Check sheet for the modelled part. Datum: model origin and axes. Units: mm. Round coordinates to 2 decimals unless told otherwise and drop trailing zeros. Answer in a Markdown table with one row per item.
from build123d import *

# Parameters (mm, degrees)
SKETCH_1_W      = 1.6
SKETCH_1_H      = 5.6
SKETCH_1_W_2    = 1.25
EXTRUDE_1_DEPTH = 100


with BuildPart() as part:
    # 草图1 → 凸台-拉伸1 (new body)
    with BuildSketch(Plane.XY):
        Polygon((-63.5, 1.710790235), (-63.5, -0.999209765), (63.5, -0.999209765), (63.5, 1.710790235), (61.9, 1.710790235), (59.4, 1.710790235), (58.15, 1.710790235), (56.03, 1.710790235), (54.78, 1.710790235), (52.66, 1.710790235), (51.41, 1.710790235), (49.29, 1.710790235), (48.04, 1.710790235), (45.92, 1.710790235), (44.67, 1.710790235), (42.55, 1.710790235), (41.3, 1.710790235), (39.18, 1.710790235), (37.93, 1.710790235), (35.81, 1.710790235), (34.56, 1.710790235), (32.44, 1.710790235), (31.19, 1.710790235), (29.07, 1.710790235), (27.82, 1.710790235), (25.7, 1.710790235), (24.45, 1.710790235), (22.33, 1.710790235), (21.08, 1.710790235), (18.96, 1.710790235), (17.71, 1.710790235), (15.59, 1.710790235), (14.34, 1.710790235), (12.22, 1.710790235), (10.97, 1.710790235), (8.85, 1.710790235), (7.6, 1.710790235), (5.48, 1.710790235), (4.23, 1.710790235), (2.11, 1.710790235), (0.86, 1.710790235), (-1.26, 1.710790235), (-2.51, 1.710790235), (-4.63, 1.710790235), (-5.88, 1.710790235), (-8, 1.710790235), (-9.25, 1.710790235), (-11.37, 1.710790235), (-12.62, 1.710790235), (-14.74, 1.710790235), (-15.99, 1.710790235), (-18.11, 1.710790235), (-19.36, 1.710790235), (-21.48, 1.710790235), (-22.73, 1.710790235), (-24.85, 1.710790235), (-26.1, 1.710790235), (-28.22, 1.710790235), (-29.47, 1.710790235), (-31.59, 1.710790235), (-32.84, 1.710790235), (-34.96, 1.710790235), (-36.21, 1.710790235), (-38.33, 1.710790235), (-39.58, 1.710790235), (-41.7, 1.710790235), (-42.95, 1.710790235), (-45.07, 1.710790235), (-46.32, 1.710790235), (-48.44, 1.710790235), (-49.69, 1.710790235), (-51.81, 1.710790235), (-53.06, 1.710790235), (-55.18, 1.710790235), (-56.43, 1.710790235), (-58.55, 1.710790235), (-59.8, 1.710790235), (-61.9, 1.710790235), align=None)
        with Locations((-62.7, 4.510790235)):
            Rectangle(SKETCH_1_W, SKETCH_1_H)
        with Locations((62.7, 4.510790235)):
            Rectangle(SKETCH_1_W, SKETCH_1_H)
        with Locations((-59.175, 4.510790235)):
            Rectangle(SKETCH_1_W_2, SKETCH_1_H)
        with Locations((58.775, 4.510790235)):
            Rectangle(SKETCH_1_W_2, SKETCH_1_H)
        with Locations((-55.805, 4.510790235)):
            Rectangle(SKETCH_1_W_2, SKETCH_1_H)
        with Locations((55.405, 4.510790235)):
            Rectangle(SKETCH_1_W_2, SKETCH_1_H)
        with Locations((-52.435, 4.510790235)):
            Rectangle(SKETCH_1_W_2, SKETCH_1_H)
        with Locations((52.035, 4.510790235)):
            Rectangle(SKETCH_1_W_2, SKETCH_1_H)
        with Locations((-49.065, 4.510790235)):
            Rectangle(SKETCH_1_W_2, SKETCH_1_H)
        with Locations((48.665, 4.510790235)):
            Rectangle(SKETCH_1_W_2, SKETCH_1_H)
        with Locations((-45.695, 4.510790235)):
            Rectangle(SKETCH_1_W_2, SKETCH_1_H)
        with Locations((45.295, 4.510790235)):
            Rectangle(SKETCH_1_W_2, SKETCH_1_H)
        with Locations((-42.325, 4.510790235)):
            Rectangle(SKETCH_1_W_2, SKETCH_1_H)
        with Locations((41.925, 4.510790235)):
            Rectangle(SKETCH_1_W_2, SKETCH_1_H)
        with Locations((-38.955, 4.510790235)):
            Rectangle(SKETCH_1_W_2, SKETCH_1_H)
        with Locations((38.555, 4.510790235)):
            Rectangle(SKETCH_1_W_2, SKETCH_1_H)
        with Locations((-35.585, 4.510790235)):
            Rectangle(SKETCH_1_W_2, SKETCH_1_H)
        with Locations((35.185, 4.510790235)):
            Rectangle(SKETCH_1_W_2, SKETCH_1_H)
        with Locations((-32.215, 4.510790235)):
            Rectangle(SKETCH_1_W_2, SKETCH_1_H)
        with Locations((31.815, 4.510790235)):
            Rectangle(SKETCH_1_W_2, SKETCH_1_H)
        with Locations((-28.845, 4.510790235)):
            Rectangle(SKETCH_1_W_2, SKETCH_1_H)
        with Locations((28.445, 4.510790235)):
            Rectangle(SKETCH_1_W_2, SKETCH_1_H)
        with Locations((-25.475, 4.510790235)):
            Rectangle(SKETCH_1_W_2, SKETCH_1_H)
        with Locations((25.075, 4.510790235)):
            Rectangle(SKETCH_1_W_2, SKETCH_1_H)
        with Locations((-22.105, 4.510790235)):
            Rectangle(SKETCH_1_W_2, SKETCH_1_H)
        with Locations((21.705, 4.510790235)):
            Rectangle(SKETCH_1_W_2, SKETCH_1_H)
        with Locations((-18.735, 4.510790235)):
            Rectangle(SKETCH_1_W_2, SKETCH_1_H)
        with Locations((18.335, 4.510790235)):
            Rectangle(SKETCH_1_W_2, SKETCH_1_H)
        with Locations((-15.365, 4.510790235)):
            Rectangle(SKETCH_1_W_2, SKETCH_1_H)
        with Locations((14.965, 4.510790235)):
            Rectangle(SKETCH_1_W_2, SKETCH_1_H)
        with Locations((-11.995, 4.510790235)):
            Rectangle(SKETCH_1_W_2, SKETCH_1_H)
        with Locations((11.595, 4.510790235)):
            Rectangle(SKETCH_1_W_2, SKETCH_1_H)
        with Locations((-8.625, 4.510790235)):
            Rectangle(SKETCH_1_W_2, SKETCH_1_H)
        with Locations((8.225, 4.510790235)):
            Rectangle(SKETCH_1_W_2, SKETCH_1_H)
        with Locations((-5.255, 4.510790235)):
            Rectangle(SKETCH_1_W_2, SKETCH_1_H)
        with Locations((4.855, 4.510790235)):
            Rectangle(SKETCH_1_W_2, SKETCH_1_H)
        with Locations((-1.885, 4.510790235)):
            Rectangle(SKETCH_1_W_2, SKETCH_1_H)
        with Locations((1.485, 4.510790235)):
            Rectangle(SKETCH_1_W_2, SKETCH_1_H)
    extrude(amount=EXTRUDE_1_DEPTH)


solid = part.part
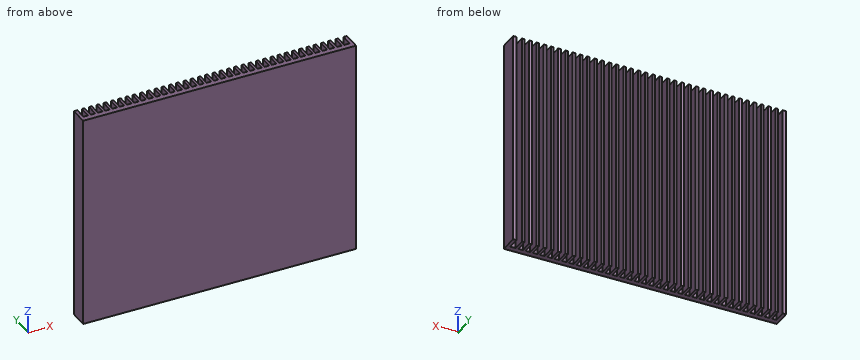
Item 1: Cross-section at A-A (y = 3). State how many separate pieces and enclosed holes the cut face has, and give its area (3 significant figures).
Result sheet:
| item | result |
|---|---|
| separate pieces | 38 |
| enclosed holes | 0 |
| area | 4,820 mm^2 |
Item 2: Depth check by flat-ended pin: P1, Ø0.6, axis at x = 16.5, z = 47.5, coming from the +Y side. Enter the tip coordinate at first touch or a pass-through.
Result sheet:
| item | result |
|---|---|
| P1 | stops at y = 1.71 |
Item 3: Scan line: line 1 (Y direction, x = -34, z = 15). Record every from-to range of solid material in increasing order. Write a range as [from, to].
Result sheet:
| item | result |
|---|---|
| line 1 | y = [-1, 1.71] |
